from build123d import *

# Parameters (mm, degrees)
SKETCH1_W          = 50.8
SKETCH1_H          = 180
BASE_FLANGE1_DEPTH = 0.7
EDGE_FLANGE1_DEPTH = 25.4
SKETCH9_W          = 25.4
SKETCH9_H          = 44.45
CUT_EXTRUDE1_DEPTH = 10
EDGE_FLANGE2_DEPTH = 50.8


# Sheet-metal steps are written as plain solids
with BuildPart() as part:
    # Sketch1 → Base-Flange1 (new body)
    with BuildSketch(Plane.XY):
        with Locations((0, -20.15)):
            Rectangle(SKETCH1_W, SKETCH1_H)
    extrude(amount=-BASE_FLANGE1_DEPTH)

    # Edge-Flange1 section (across the edge) → Edge-Flange1 (add)
    with BuildSketch(Plane(origin=(-26.4, -110.15, -0.7), x_dir=(1, 0, 0), z_dir=(0, 1, 0))):
        with BuildLine():
            Line((-0.7, 1), (-0.7, 24.7))
            Line((-0.7, 24.7), (0, 24.7))
            Line((0, 24.7), (0, 1))
            ThreePointArc((0, 1), (0.292893219, 0.292893219), (1, 0))
            Line((1, 0), (1, -0.7))
            ThreePointArc((1, -0.7), (-0.202081528, -0.202081528), (-0.7, 1))
        make_face()
    extrude(amount=EDGE_FLANGE1_DEPTH)

    # Sketch9 → Cut-Extrude1 (cut)
    with BuildSketch(Plane.XY):
        with Locations((12.7, -87.925)):
            Rectangle(SKETCH9_W, SKETCH9_H)
    extrude(amount=-CUT_EXTRUDE1_DEPTH, mode=Mode.SUBTRACT)

    # Edge-Flange2 section (across the edge) → Edge-Flange2 (add)
    with BuildSketch(Plane(origin=(-25.4, 70.264213562, -0.7), x_dir=(0, -0.7071067811865438, -0.7071067811865512), z_dir=(1, 0, 0))):
        with BuildLine():
            Line((-0.7, 0.414213562), (-0.7, 75.910050506))
            Line((-0.7, 75.910050506), (0, 75.910050506))
            Line((0, 75.910050506), (0, 0.414213562))
            ThreePointArc((0, 0.414213562), (0.076120467, 0.03153013), (0.292893219, -0.292893219))
            Line((0.292893219, -0.292893219), (-0.202081528, -0.787867966))
            ThreePointArc((-0.202081528, -0.787867966), (-0.570595205, -0.236348273), (-0.7, 0.414213562))
        make_face()
    extrude(amount=EDGE_FLANGE2_DEPTH)


solid = part.part
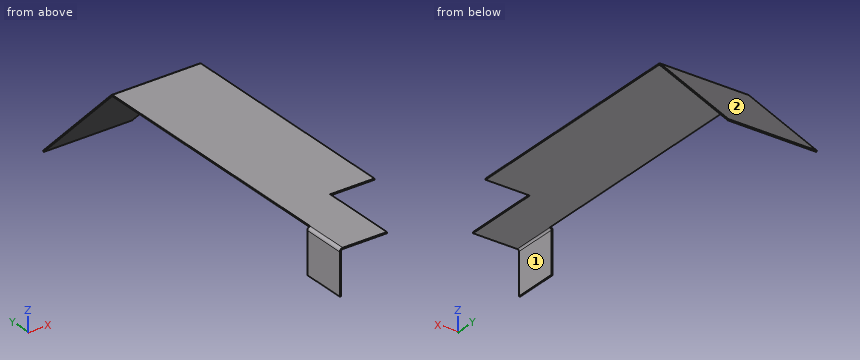
CAD build for the part. Positions are in the model's coordinates, mm. Face numbers are marked on the shaded views. A direction names the side the tool comes from. Round coordinates to 2 decimals unless told otherwise and drop trailing zeros. Write each loop counter-clockwise with the first axis right and the second up, starting at its lowest first coordinate (ties: lowest second). Pieces come first, ordered by that corner, then holes. Notation, with made-up numbers: M 35,88.5 L 71,88.5 A30 ccw 71,122.5 Z; hole C 71.25,-17.5 d4. An arc over 180 degrees is marked long. Put each result on its own line as item: value. Start each with the question number.
1) Saw through at D-D, the plane y = -3. Write the cut outline in (x, z), and give its area (3 significant figures).
2) Saw through at B-B, the plane z = -16.5. Write the cut outline in (x, y).
3) Saw through at A-A, the plane x = -15.5. Write the cut outline in (y, z).
4) Drill centre lines: probe 1 along Z at (x, y) = (-4, -68.5); probe 2 along Y at (x, z) = (3.5, -35.5); probe 3 along Y at (x, z) = (-22.5, -34). Where is each one in solid material? Low to high. Write a range as [from, to].
5) Pin check, flat tips, straight feed: pin 1 Ø8 at (x, z) = (13.5, -46) entering from -Y; pin 2 Ø2 at (x, y) = (17.5, -66.5) entering from -Z; pin 3 Ø0.5 at (x, z) = (-26.5, -7.5) entering from +Y. Stop position of each tip, or through.
6) Saw through at C-C, the plane x = 12. Write the cut outline in (y, z), and give its area (3 significant figures).
7) 3-axis set-ups, long thin cutter, end or side, ignore diameter. For the marked faces 1 and 2: which of +Z, -Z, +X, -X, +Y, -Y reach the whole face in a straight line?
Resolved:
1. outline: M -25.4,-0.7 L 25.4,-0.7 L 25.4,0 L -25.4,0 Z
1. area: 35.6 mm²
2. outline: M -27.1,-110.15 L -26.4,-110.15 L -26.4,-84.75 L -27.1,-84.75 Z; M -25.4,86.06 L 25.4,86.06 L 25.4,87.05 L -25.4,87.05 Z
3. outline: M -110.15,-0.7 L 69.85,-0.7 A1 cw 70.56,-0.99 L 123.94,-54.38 L 124.44,-53.88 L 71.05,-0.5 A1.7 ccw 69.85,0 L -110.15,0 Z
4. probe 1: [-0.7, 0]
4. probe 2: [105.06, 106.05]
4. probe 3: [103.56, 104.55]
5. pin 1: y = 111.56
5. pin 2: z = -0.7
5. pin 3: y = -84.75
6. outline: M -65.7,-0.7 L 69.85,-0.7 A1 cw 70.56,-0.99 L 123.94,-54.38 L 124.44,-53.88 L 71.05,-0.5 A1.7 ccw 69.85,0 L -65.7,0 Z
6. area: 148 mm²
7. face 1: -Z, +X, +Y, -Y
7. face 2: +Z, +X, -X, +Y
